```python
from build123d import *

# Parameters (mm, degrees)
FILLET1_R = 2


with BuildPart() as part:
    # Sketch1 → Revolve1 (revolve)
    with BuildSketch(Plane(origin=(0, 0, 0), x_dir=(0, 0, -1), z_dir=(1, 0, 0)), mode=Mode.PRIVATE) as revolve1_sk:
        with BuildLine():
            Line((0, 0), (0, -12.7))
            Line((0, -12.7), (5, -12.7))
            Line((5, -12.7), (5, -19))
            Line((5, -19), (38, -19))
            Line((38, -19), (38, -18))
            Line((38, -18), (34.517434791, -14.517434791))
            ThreePointArc((34.517434791, -14.517434791), (37.117181053, -7.464652928), (38, 0))
            Line((38, 0), (6, 0))
            Line((6, 0), (0, 0))
        make_face()
    revolve(revolve1_sk.sketch.rotate(Axis((0, 0, 0), (0, 0, -1)), 270), axis=Axis((0, 0, 0), (0, 0, -1)))

    # Fillet1
    fillet1_edges = [part.edges().sort_by_distance(p)[0] for p in [
        (-19, 0, -5),
    ]]
    fillet(fillet1_edges, radius=FILLET1_R)


solid = part.part
```
Can you work these out from the model? Positions are in its coordinate system, mm. A direction names the side the tool comes from. Round coordinates to 2 decimals unless told otherwise and drop trailing zeros. Loops run counter-clockwise (first coordinate to the right, second up) from the corner with the lowest first, then second, coordinate; pieces in that order, holes last. Notation, with made-up numbers: (45.25, 14.25) -> (82.25, 14.25) arc R28 cw to (82.25, 41.25) -> close; hole circle Ø6 at (53, -14). An arc over 180 degrees is marked (long way). One line per item, written item: value. Start each with the question number.
1. For faces 1 (the flat face through (13, 1, -5)), 2 (the flat face through (7, 17, -38)), which set-ups out of +Z, -Z, +X, -X, +Y, -Y let a thin tool reach every point of the face, with its end or its side?
2. If we section it at A-A, the plane x = 0: Write out the boundary of the cut face in (y, z), then the cut area to 3 significant figures.
3. If we mould it in two halves opening along Y, with no side actions, what happens to faces 3 (the conical face through (13.57, 5.63, -34.69)), 4 (the flat face through (0, 0, 0)), 5 (the cylindrical face through (-10.1, 7.7, -2.5))? For each: pulls with the +Y half, pulls with the -Y half, needs draft (parallel to the pull), parting line crosses it, or undercut.
4. If we section it at C-C, the plane z = -17.5: Write out the boundary of the cut face in (x, y).
5. For pin 1 (6 mm diameter, centred on x = 3.5, z = -31, fed in from +Y); pin 2 (12 mm diameter, centred on y = -7.5, z = -21.5, fed in from +X); pin 3 (8 mm diameter, centred on x = 11, y = -5.5, fed in from -Z), each with a flat end and sliding along its axis, tell me the tip position at first contact or that it passes through.
6. If I drill on probe 1 along Y at (x, z) = (-0.5, -31); probe 2 along Z at (x, y) = (6.5, 3); probe 3 along Z at (x, y) = (2, 17.5), over which ranges is the centre line in solid material (lowest first)?
Calculated:
1. face 1: +Z
1. face 2: -Z, +X, -X, +Y, -Y
2. outline: (-19, -38) -> (-18, -38) -> (-14.52, -34.52) arc R32 ccw to (14.52, -34.52) -> (18, -38) -> (19, -38) -> (19, -7) arc R2 ccw to (17, -5) -> (12.7, -5) -> (12.7, 0) -> (-12.7, 0) -> (-12.7, -5) -> (-17, -5) arc R2 ccw to (-19, -7) -> close
2. area: 1,330 mm²
3. face 3: undercut
3. face 4: needs draft
3. face 5: parting line crosses it
4. outline: circle Ø38 at (0, 0)
5. pin 1: stops at y = 18.99
5. pin 2: stops at x = 18.94
5. pin 3: stops at z = -36.91
6. probe 1: y = -18.99 to 18.99
6. probe 2: z = -37.19 to 0
6. probe 3: z = -37.61 to -5.1
